Can you work these out from the model? Positions are in its coordinate system, mm. A direction names the side the tool comes from. Round coordinates to 2 decimals unless told otherwise and drop trailing zeros. Write each loop counter-clockwise with the first axis right and the second up, starting at its lowest first coordinate (ties: lowest second). Pieces come first, ordered by that corner, then holes. Notation, with made-up numbers: M 86.25,51 L 129.25,51 A6 cw 129.25,61 Z; hole C -35.5,86.5 d1. An arc over 180 degrees is marked long. Answer in a Markdown table with one row per item. Add a question column.
(1) If I drill on probe 1 along Y at (x, z) = (8.5, 7); probe 2 along Y at (x, z) = (16, -17); probe 3 along Y at (x, z) = (5.5, 18), over which ranges is the centre line in solid material (lowest first)?
(2) For faces 4 (the face through (0.03, 1.48, -17.75)), 5 (the face through (7.509, 104.844, 23.846)), 6 (the face through (0.33, 44.038, -7.493)), which set-ups out of +Z, -Z, +X, -X, +Y, -Y let a thin tool reach every point of the face, with its end or its side?
(3) Suppose I cut it at A-A, the plane z = 0. Count the separate pieces of the cut face and the enclosed holes in it, then the cut area to 3 significant figures.
(4) Suppose I cut it at B-B, the plane y = 9. Write out the boundary of the cut face in (x, z), then the cut area to 3 significant figures.
(5) If we mould it in two halves opening along Z, with no side actions, what happens to faces 1 (the face through (-1.25, 2, 13)), 2 (the face through (-8, 3, 8)), 3 (the face through (-19.524, 0.493, -4.336))? For each: released by +Z, released by -Z, zero draft, split by the parting line, or undercut.
(6) I'm going to push flat-ended pins straight in: pin 1 (3.5 mm diameter, centred on y = 2, z = -14.5, fed in from -X); pin 2 (12 mm diameter, centred on y = 57.5, z = 11, fed in from +X); pin 3 (8 mm diameter, centred on y = 56.5, z = 8, fed in from -X). Where does each tip first touch, or does it pass through?
from build123d import *

# Parameters (mm, degrees)
SKETCH1_R           = 20
BOSS_EXTRUDE1_DEPTH = 3
SKETCH2_R           = 7.5
BOSS_EXTRUDE2_DEPTH = 100
SKETCH3_R           = 25
BOSS_EXTRUDE3_DEPTH = 2
FILLET3_R           = 20
FILLET4_R           = 2
FILLET6_R           = 3
CUT_EXTRUDE1_REACH  = 112.793
FILLET8_R           = 2


with BuildPart() as part:
    # Sketch1 → Boss-Extrude1 (new body)
    with BuildSketch(Plane(origin=(0, 0, 0), x_dir=(1, 0, 0), z_dir=(0, 1, 0))):
        with Locations(Location((0, 0, 0), (0, 0, 270))):
            Circle(SKETCH1_R)
    extrude(amount=BOSS_EXTRUDE1_DEPTH)

    # Sketch2 → Boss-Extrude2 (add)
    with BuildSketch(Plane(origin=(0, 3, 0), x_dir=(1, 0, 0), z_dir=(0, 1, 0))):
        with Locations(Location((0, 0, 0), (0, 0, 270))):
            Circle(SKETCH2_R)
    extrude(amount=BOSS_EXTRUDE2_DEPTH)

    # Sketch3 → Boss-Extrude3 (add)
    with BuildSketch(Plane(origin=(0, 103, 0), x_dir=(1, 0, 0), z_dir=(0, 1, 0))):
        with Locations(Location((0, 0, 0), (0, 0, 270))):
            Circle(SKETCH3_R)
    extrude(amount=BOSS_EXTRUDE3_DEPTH)

    # Fillet3
    # the kernel refuses this fillet: 20 mm, written as the material it adds along each edge
    with BuildSketch(Plane(origin=(0, 103, 0), x_dir=(0, 0, 1), z_dir=(-1, 0, 0))) as fillet3_piece_1:
        with BuildLine():
            CenterArc((27.5, -19.843134833), FILLET3_R, 97.180755781, 82.819244219)
            Line((7.5, -19.843134833), (7.1, -19.843134833))
            Line((7.1, -19.843134833), (7.1, 0))
            Line((7.1, 0), (7.5, 0.4))
            ThreePointArc((7.5, 0.4), (16.25, 0.4), (24.95, 0.396862697))
            Line((24.95, 0.396862697), (25, 0))
        make_face()
    revolve(axis=Axis((0, 103, 0), (0, 1, 0)))

    # Fillet4
    fillet4_edges = [part.edges().sort_by_distance(p)[0] for p in [
        (0, 103, -25),
    ]]
    fillet(fillet4_edges, radius=FILLET4_R)

    # Fillet6
    fillet6_edges = [part.edges().sort_by_distance(p)[0] for p in [
        (0, 3, -7.5),
    ]]
    fillet(fillet6_edges, radius=FILLET6_R)

    # Sketch4 → Cut-Extrude1 (cut, up to next)
    with BuildSketch(Plane.XZ, mode=Mode.PRIVATE) as cut_extrude1_sk1:
        with BuildLine():
            Line((-1.25, -16.5), (-1.25, -9.5))
            ThreePointArc((-1.25, -9.5), (0, -8.25), (1.25, -9.5))
            Line((1.25, -9.5), (1.25, -16.5))
            ThreePointArc((1.25, -16.5), (0, -17.75), (-1.25, -16.5))
        make_face()
    cut_extrude1_tool1 = extrude(cut_extrude1_sk1.sketch, amount=-CUT_EXTRUDE1_REACH, mode=Mode.PRIVATE) & part.part
    # Sketch4 → Cut-Extrude1 (cut, up to next)
    with BuildSketch(Plane.XZ, mode=Mode.PRIVATE) as cut_extrude1_sk2:
        with BuildLine():
            Line((-16.5, 1.25), (-9.5, 1.25))
            ThreePointArc((-9.5, 1.25), (-8.25, 0), (-9.5, -1.25))
            Line((-9.5, -1.25), (-16.5, -1.25))
            ThreePointArc((-16.5, -1.25), (-17.75, 0), (-16.5, 1.25))
        make_face()
    cut_extrude1_tool2 = extrude(cut_extrude1_sk2.sketch, amount=-CUT_EXTRUDE1_REACH, mode=Mode.PRIVATE) & part.part
    # Sketch4 → Cut-Extrude1 (cut, up to next)
    with BuildSketch(Plane.XZ, mode=Mode.PRIVATE) as cut_extrude1_sk3:
        with BuildLine():
            Line((1.25, 16.5), (1.25, 9.5))
            ThreePointArc((1.25, 9.5), (0, 8.25), (-1.25, 9.5))
            Line((-1.25, 9.5), (-1.25, 16.5))
            ThreePointArc((-1.25, 16.5), (0, 17.75), (1.25, 16.5))
        make_face()
    cut_extrude1_tool3 = extrude(cut_extrude1_sk3.sketch, amount=-CUT_EXTRUDE1_REACH, mode=Mode.PRIVATE) & part.part
    # Sketch4 → Cut-Extrude1 (cut, up to next)
    with BuildSketch(Plane.XZ, mode=Mode.PRIVATE) as cut_extrude1_sk4:
        with BuildLine():
            Line((16.5, -1.25), (9.5, -1.25))
            ThreePointArc((9.5, -1.25), (8.25, 0), (9.5, 1.25))
            Line((9.5, 1.25), (16.5, 1.25))
            ThreePointArc((16.5, 1.25), (17.75, 0), (16.5, -1.25))
        make_face()
    cut_extrude1_tool4 = extrude(cut_extrude1_sk4.sketch, amount=-CUT_EXTRUDE1_REACH, mode=Mode.PRIVATE) & part.part
    add(cut_extrude1_tool1.solids().sort_by_distance((0, 0, -13))[0], mode=Mode.SUBTRACT)
    add(cut_extrude1_tool2.solids().sort_by_distance((-13, 0, 0))[0], mode=Mode.SUBTRACT)
    add(cut_extrude1_tool3.solids().sort_by_distance((0, 0, 13))[0], mode=Mode.SUBTRACT)
    add(cut_extrude1_tool4.solids().sort_by_distance((13, 0, 0))[0], mode=Mode.SUBTRACT)

    # Fillet8
    fillet8_edges = [part.edges().sort_by_distance(p)[0] for p in [
        (0, 3, -20),
    ]]
    fillet(fillet8_edges, radius=FILLET8_R)


solid = part.part
Calculated:
| question | item | result |
|---|---|---|
| 1 | probe 1 | 0 to 3, 94.48 to 105 |
| 1 | probe 2 | 102.72 to 105 |
| 1 | probe 3 | 0 to 2.82, 101.18 to 105 |
| 2 | face 4 | -Y |
| 2 | face 5 | +Y, -Y |
| 2 | face 6 | none |
| 3 | separate pieces | 3 |
| 3 | enclosed holes | 0 |
| 3 | area | 1,830 mm² |
| 4 | outline | C 0,0 d15 |
| 4 | area | 177 mm² |
| 5 | face 1 | undercut |
| 5 | face 2 | zero draft |
| 5 | face 3 | split by the parting line |
| 6 | pin 1 | x = -15.27 |
| 6 | pin 2 | x = 5.59 |
| 6 | pin 3 | x = -6.34 |
